Autodesk Inventor part; units mm, degrees
ref_plane "YZ Plane" through (0, 0, 0) normal (1, 0, 0) x (0, 1, 0)
ref_plane "XZ Plane" through (0, 0, 0) normal (0, 1, 0) x (-1, 0, 0)
ref_plane "XY Plane" through (0, 0, 0) normal (0, 0, 1) x (1, 0, 0)
sketch "スケッチ1" plane through (0, 0, 0) normal (0, 1, 0) x (-1, 0, 0)
  circle A0 centre (0, 0) radius 2
  dimension "d0" = 4
extrude "押し出し1" add sketch "スケッチ1" along normal blind 22.56
sketch "スケッチ2" plane through (0, 22.56, 0) normal (0, 1, 0) x (1, 0, 0)
  point P0 (0, 0)
hole "穴1" at (0, 22.56, 0) direction (0, -1, 0) diameter 2 end through all countersink diameter 3 countersink angle 90
sketch "スケッチ3" plane through (0, 0, 0) normal (0, -1, 0) x (1, 0, 0)
  point P0 (0, 0)
hole "穴2" at (0, 0, 0) direction (0, 1, 0) diameter 2 end through all countersink diameter 3 countersink angle 90
properties part number "shaft" material "鉄、鋳鉄"
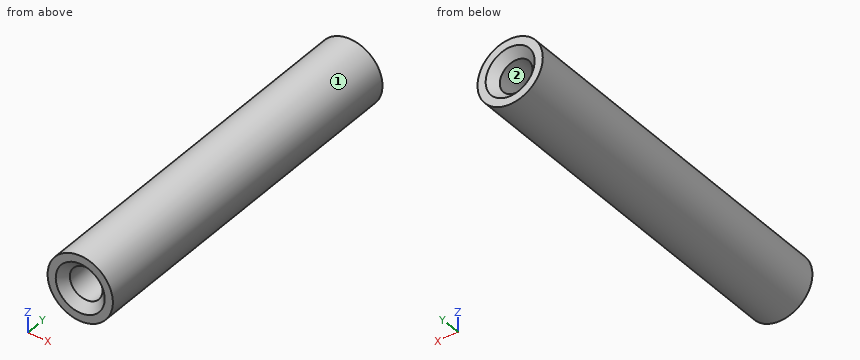
Here's how the part is built. I have some questions about the finished solid (model axes, mm). Face numbers are marked on the shaded views. Coordinates: 2 decimals unless noted, no trailing zeros. Order: outer loops, then holes, each group sorted by start corner. A loop starts at its lowest first (then second) coordinate and runs counter-clockwise, first axis right, second up.
Item 1: I need wall thicknesses on line 1 (X direction, y = 1, z = -0.1); line 2 (X direction, y = 1.5, z = -0.85). Which ranges of each line are inside material? Lowest first, please.
Result sheet:
line 1: x = -2 to -0.99, 0.99 to 2
line 2: x = -1.81 to -0.53, 0.53 to 1.81
Item 2: If we section it at B-B on z = 0: List the corners of the cut face in (x, y) for me, plus the area to 3 significant figures.
Result sheet:
outline: (-2, 0) - (-1.5, 0) - (-1, 0.5) - (-1, 22.06) - (-1.5, 22.56) - (-2, 22.56) - close; (1, 0.5) - (1.5, 0) - (2, 0) - (2, 22.56) - (1.5, 22.56) - (1, 22.06) - close
area: 44.6 mm2
Item 3: If we mould it in two halves opening along Z, with no side actions, what happens to the marked faces 1 and 2? For each: +Z half, -Z half, draft (parallel to the pull), parting line (faces both ways), or undercut.
Result sheet:
face 1: parting line
face 2: undercut
Item 4: If we section it at C-C on y = 18.25: List the corners of the cut face in (x, z) for me.
Result sheet:
outline: circle Ø4 at (0, 0); hole circle Ø2 at (0, 0)
Item 5: If we section it at A-A on x = 0: List the corners of the cut face in (y, z) for me, plus the area to 3 significant figures.
Result sheet:
outline: (0, -2) - (22.56, -2) - (22.56, -1.5) - (22.06, -1) - (0.5, -1) - (0, -1.5) - close; (0, 1.5) - (0.5, 1) - (22.06, 1) - (22.56, 1.5) - (22.56, 2) - (0, 2) - close
area: 44.6 mm2
Item 6: If we section it at D-D on x = 1.7: List the corners of the cut face in (y, z) for me.
Result sheet:
outline: (0, -1.05) - (22.56, -1.05) - (22.56, 1.05) - (0, 1.05) - close
